Autodesk Inventor part; units mm, degrees
ref_plane "YZ Plane" through (0, 0, 0) normal (1, 0, 0) x (0, 1, 0)
ref_plane "XZ Plane" through (0, 0, 0) normal (0, 1, 0) x (-1, 0, 0)
ref_plane "XY Plane" through (0, 0, 0) normal (0, 0, 1) x (1, 0, 0)
sketch "Sketch1" plane through (0, 0, 0) normal (0, 1, 0) x (-1, 0, 0)
  line L0 (-60.452, -60.452) -> (60.452, -60.452)
  line L1 (60.452, -60.452) -> (60.452, 60.452)
  line L2 (60.452, 60.452) -> (-60.452, 60.452)
  line L3 (-60.452, 60.452) -> (-60.452, -60.452)
  line L4 (-60.452, -60.452) -> (60.452, 60.452) construction
  line L5 (60.452, -60.452) -> (-60.452, 60.452) construction
  point P0 (0, 0)
  dimension "d0" = 120.904
  dimension "d1" = 120.904
extrude "Extrusion1" add sketch "Sketch1" along normal blind 2.54
sketch "Sketch2" plane through (0, 2.54, 0) normal (0, 1, 0) x (1, 0, 0)
  line L0 (60.452, 60.452) -> (-60.452, 60.452)
  line L1 (60.452, -60.452) -> (-60.452, -60.452)
  line L2 (-60.452, -60.452) -> (-60.452, 60.452)
  line L3 (-60.452, 60.452) -> (60.452, 60.452)
  line L4 (60.452, 60.452) -> (60.452, -60.452)
  line L5 (60.452, -60.452) -> (-60.452, 60.452) construction
  line L6 (-60.452, -60.452) -> (60.452, 60.452) construction
  line L7 (59.182, -59.182) -> (-59.182, -59.182)
  line L8 (-59.182, -59.182) -> (-59.182, 59.182)
  line L9 (-59.182, 59.182) -> (59.182, 59.182)
  line L10 (59.182, 59.182) -> (59.182, -59.182)
  line L11 (59.182, -59.182) -> (-59.182, 59.182) construction
  line L12 (-59.182, -59.182) -> (59.182, 59.182) construction
  point P0 (0, 0)
  dimension "d4" = 118.364
  dimension "d5" = 118.364
extrude "Extrusion2" add sketch "Sketch2" along normal blind 82.804
sketch "Sketch3" plane through (0, 2.54, 0) normal (0, 1, 0) x (1, 0, 0)
  circle A0 centre (0, -25.4) radius 2.0828
  circle A1 centre (0, 25.4) radius 2.0828
  point P0 (0, 0)
  dimension "d10" = 4.1656
  dimension "d11" = 4.1656
extrude "Extrusion3" cut sketch "Sketch3" against normal through all
properties part number "546-1550Z137-4.8x4.8-Enclosure"
Input: part model. Units: mm. Frame: model coordinates. A direction names the side the tool comes from. Give positions to 0.01 mm unless a question says otherwise; leave off trailing zeros. Write each loop counter-clockwise with the first axis right and the second up, starting at its lowest first coordinate (ties: lowest second). Pieces come first, ordered by that corner, then holes. Notation, with made-up numbers: (42, -33) - (78, -33) arc R23 cw to (78, -17) - close; hole circle Ø10 at (-25.5, -33). An arc over 180 degrees is marked (long way). Write item = value, one per line. Start each with the question number.
1. Section query C-C, the plane x = 0. Output: boundary loops of the cut face in (y, z), then the cut area to 3 significant figures.
2. Access query for faces 1 (the cylindrical face through (0.96, 1.29, 27.25)), 2 (the flat face through (-1, 43, -59.182)). Directions: +Z, -Z, +X, -X, +Y, -Y. A direction counts if a zero-diameter tool reaches every point of the face in a straight line with its end or side. Return the directions, or none.
3. Ray query, L1, parallel to Z at x = 0, y = 1.85; L2, parallel to X at y = 26, z = 39; L3, parallel to X at y = 1.1, z = -25.4. Return the intervals inside material, ascending.
4. Section query B-B, the plane y = 28. Output: boundary loops of the cut face in (x, z), then the cut area to 3 significant figures.
5. Section query A-A, the plane z = -25.4. Output: boundary loops of the cut face in (x, y).
6. First-contact query: pin 1 Ø10 at (x, z) = (-36.5, -10.5) entering from +Y; pin 2 Ø2 at (x, z) = (-3, 20.5) entering from -Y. Flat tips, straight axial feed; report the tip coordinate or a pass-through.
7. Mould query, pull axis X, two halves, no side actions, for faces 3 (the flat face through (-59.182, 43, 1)), 4 (the flat face through (60.452, 42, 1)), 5 (the flat face through (-1, 42, 60.452)). Classes: released by +X, released by -X, zero draft, split by the parting line, or undercut.
8. Section query D-D, the plane z = 9.5. Output: boundary loops of the cut face in (x, y), then the cut area to 3 significant figures.
Check sheet entries:
q1.outline = (0, -60.45) - (85.34, -60.45) - (85.34, -59.18) - (2.54, -59.18) - (2.54, -27.48) - (0, -27.48) - close; (0, -23.32) - (2.54, -23.32) - (2.54, 23.32) - (0, 23.32) - close; (0, 27.48) - (2.54, 27.48) - (2.54, 59.18) - (85.34, 59.18) - (85.34, 60.45) - (0, 60.45) - close
q1.area = 496 mm2
q2.face_1 = +Y, -Y
q2.face_2 = +Y
q3.L1 = -60.45 to -27.48, -23.32 to 23.32, 27.48 to 60.45
q3.L2 = -60.45 to -59.18, 59.18 to 60.45
q3.L3 = -60.45 to -2.08, 2.08 to 60.45
q4.outline = (-60.45, -60.45) - (60.45, -60.45) - (60.45, 60.45) - (-60.45, 60.45) - close; hole (-59.18, -59.18) - (59.18, -59.18) - (59.18, 59.18) - (-59.18, 59.18) - close
q4.area = 608 mm2
q5.outline = (-60.45, 0) - (-2.08, 0) - (-2.08, 2.54) - (-59.18, 2.54) - (-59.18, 85.34) - (-60.45, 85.34) - close; (2.08, 0) - (60.45, 0) - (60.45, 85.34) - (59.18, 85.34) - (59.18, 2.54) - (2.08, 2.54) - close
q6.pin_1 = 2.54
q6.pin_2 = 0
q7.face_3 = undercut
q7.face_4 = released by +X
q7.face_5 = zero draft
q8.outline = (-60.45, 0) - (60.45, 0) - (60.45, 85.34) - (59.18, 85.34) - (59.18, 2.54) - (-59.18, 2.54) - (-59.18, 85.34) - (-60.45, 85.34) - close
q8.area = 517 mm2
